Study the drawing (mm; zero at the part's minimum x, y, z) and answer. Coordinates: 2 decimals unless noted, no trailing zeros. Order: outer loops, then holes, each group sorted by start corner. A loop starts at its lowest first (then second) coordinate and runs counter-clockwise, first axis right, second up. Notation, with made-up numbers: (17, 18) - (51, 18) arc R18 cw to (51, 34) - close; hole circle Ø5 at (-4, 26.25). An arc over 180 degrees is marked (long way). Write item = value, one per line.
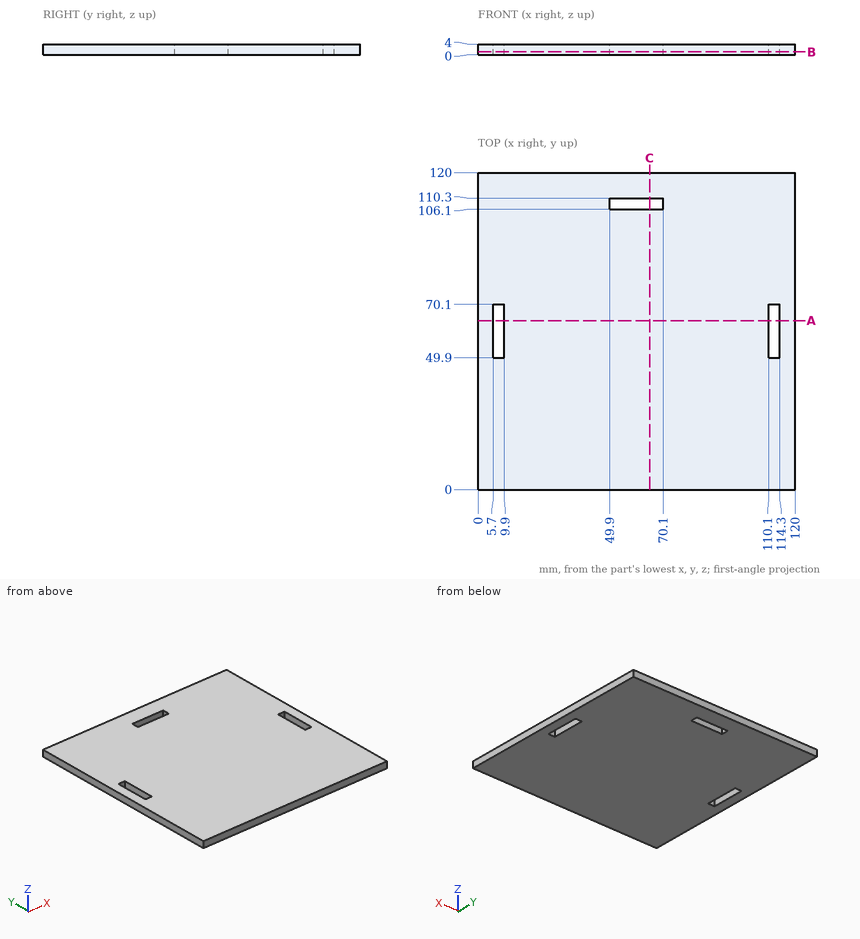
1) The part is cut by section C-C (x = 65). Determine the outline of the cut face in (y, z), and give its area (3 significant figures).
Returned:
outline = (0, 0) - (106.1, 0) - (106.1, 4) - (0, 4) - close; (110.3, 0) - (120, 0) - (120, 4) - (110.3, 4) - close
area = 463 mm^2
2) The part is cut by section A-A (y = 64). Determine the outline of the cut face in (x, z), and give its area (3 significant figures).
Returned:
outline = (0, 0) - (5.7, 0) - (5.7, 4) - (0, 4) - close; (9.9, 0) - (110.1, 0) - (110.1, 4) - (9.9, 4) - close; (114.3, 0) - (120, 0) - (120, 4) - (114.3, 4) - close
area = 446 mm^2
3) A flat-ended cylindrical pin translates along its axis: pin 1 Ø2 at (x, z) = (112.5, 2) entering from -Y. Find the tip coordinate at first contact, or state that the pin passes through.
Returned:
pin_1 = 0
4) The part is cut by section B-B (z = 1). Determine the outline of the cut face in (x, y).
Returned:
outline = (0, 0) - (120, 0) - (120, 120) - (0, 120) - close; hole (5.7, 49.9) - (9.9, 49.9) - (9.9, 70.1) - (5.7, 70.1) - close; hole (49.9, 106.1) - (70.1, 106.1) - (70.1, 110.3) - (49.9, 110.3) - close; hole (110.1, 49.9) - (114.3, 49.9) - (114.3, 70.1) - (110.1, 70.1) - close
5) Straight lines are drawn through the part: line 1 along X through (y, z) = (57.5, 3.05); line 2 along Y through (x, z) = (113.5, 0.3); line 3 along Y through (x, z) = (50, 2.9). For each, find the intervals that lie inside material, in ascending order. Write a range as from..to.
Returned:
line_1 = 0..5.7, 9.9..110.1, 114.3..120
line_2 = 0..49.9, 70.1..120
line_3 = 0..106.1, 110.3..120
